For this review, take the finished solid that the model builds, in its own axes (mm). Face numbers are marked on the shaded views. A direction names the side the tool comes from. Coordinates: 2 decimals unless noted, no trailing zeros. Loops run counter-clockwise (first coordinate to the right, second up) from the corner with the lowest first, then second, coordinate; pieces in that order, holes last. Notation, with made-up numbers: M 10,36 L 60,36 A12 cw 60,49 Z; hole C -7,37 d10. An arc over 180 degrees is marked long. Put each result on its own line as item: value.
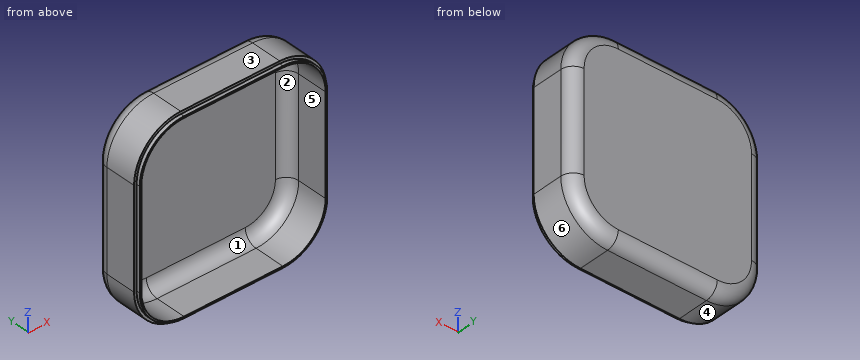
```python
from build123d import *

# Parameters (mm, degrees)
F1_DEPTH = 1.3
F2_DEPTH = 14
F4_DEPTH = 1.2
F5_R     = 4
F6_R     = 4


with BuildPart() as f1:
    # F0 (on Front) → F1 (new body)
    with BuildSketch(Plane.XZ):
        with BuildLine():
            Line((15.9, 30.9), (-15.9, 30.9))
            ThreePointArc((-15.9, 30.9), (-26.506602, 26.506602), (-30.9, 15.9))
            Line((-30.9, 15.9), (-30.9, -15.9))
            ThreePointArc((-30.9, -15.9), (-26.506602, -26.506602), (-15.9, -30.9))
            Line((-15.9, -30.9), (15.9, -30.9))
            ThreePointArc((15.9, -30.9), (26.506602, -26.506602), (30.9, -15.9))
            Line((30.9, -15.9), (30.9, 15.9))
            ThreePointArc((30.9, 15.9), (26.506602, 26.506602), (15.9, 30.9))
        make_face()
        with BuildLine():
            ThreePointArc((-29.6, 15.9), (-25.587363, 25.587363), (-15.9, 29.6))
            Line((-15.9, 29.6), (15.9, 29.6))
            ThreePointArc((15.9, 29.6), (25.587363, 25.587363), (29.6, 15.9))
            Line((29.6, 15.9), (29.6, -15.9))
            ThreePointArc((29.6, -15.9), (25.587363, -25.587363), (15.9, -29.6))
            Line((15.9, -29.6), (-15.9, -29.6))
            ThreePointArc((-15.9, -29.6), (-25.587363, -25.587363), (-29.6, -15.9))
            Line((-29.6, -15.9), (-29.6, 15.9))
        make_face(mode=Mode.SUBTRACT)
        with BuildLine():
            Line((15.9, 29.6), (-15.9, 29.6))
            ThreePointArc((-15.9, 29.6), (-25.587363, 25.587363), (-29.6, 15.9))
            Line((-29.6, 15.9), (-29.6, -15.9))
            ThreePointArc((-29.6, -15.9), (-25.587363, -25.587363), (-15.9, -29.6))
            Line((-15.9, -29.6), (15.9, -29.6))
            ThreePointArc((15.9, -29.6), (25.587363, -25.587363), (29.6, -15.9))
            Line((29.6, -15.9), (29.6, 15.9))
            ThreePointArc((29.6, 15.9), (25.587363, 25.587363), (15.9, 29.6))
        make_face()
    extrude(amount=F1_DEPTH)

    # F0 (on Front) → F2 (join)
    with BuildSketch(Plane.XZ):
        with BuildLine():
            Line((15.9, 30.9), (-15.9, 30.9))
            ThreePointArc((-15.9, 30.9), (-26.506602, 26.506602), (-30.9, 15.9))
            Line((-30.9, 15.9), (-30.9, -15.9))
            ThreePointArc((-30.9, -15.9), (-26.506602, -26.506602), (-15.9, -30.9))
            Line((-15.9, -30.9), (15.9, -30.9))
            ThreePointArc((15.9, -30.9), (26.506602, -26.506602), (30.9, -15.9))
            Line((30.9, -15.9), (30.9, 15.9))
            ThreePointArc((30.9, 15.9), (26.506602, 26.506602), (15.9, 30.9))
        make_face()
        with BuildLine():
            ThreePointArc((-29.6, 15.9), (-25.587363, 25.587363), (-15.9, 29.6))
            Line((-15.9, 29.6), (15.9, 29.6))
            ThreePointArc((15.9, 29.6), (25.587363, 25.587363), (29.6, 15.9))
            Line((29.6, 15.9), (29.6, -15.9))
            ThreePointArc((29.6, -15.9), (25.587363, -25.587363), (15.9, -29.6))
            Line((15.9, -29.6), (-15.9, -29.6))
            ThreePointArc((-15.9, -29.6), (-25.587363, -25.587363), (-29.6, -15.9))
            Line((-29.6, -15.9), (-29.6, 15.9))
        make_face(mode=Mode.SUBTRACT)
    extrude(amount=F2_DEPTH)

    # F3 (on face) → F4 (join)
    with BuildSketch(Plane.XZ.offset(14)):
        with BuildLine():
            Line((15.9, 30.1), (-15.9, 30.1))
            ThreePointArc((-15.9, 30.1), (-25.940916, 25.940916), (-30.1, 15.9))
            Line((-30.1, 15.9), (-30.1, -15.9))
            ThreePointArc((-30.1, -15.9), (-25.940916, -25.940916), (-15.9, -30.1))
            Line((-15.9, -30.1), (15.9, -30.1))
            ThreePointArc((15.9, -30.1), (25.940916, -25.940916), (30.1, -15.9))
            Line((30.1, -15.9), (30.1, 15.9))
            ThreePointArc((30.1, 15.9), (25.940916, 25.940916), (15.9, 30.1))
        make_face()
        with BuildLine():
            Line((15.9, -29.6), (-15.9, -29.6))
            ThreePointArc((-15.9, -29.6), (-25.587363, -25.587363), (-29.6, -15.9))
            Line((-29.6, -15.9), (-29.6, 15.9))
            ThreePointArc((-29.6, 15.9), (-25.587363, 25.587363), (-15.9, 29.6))
            Line((-15.9, 29.6), (15.9, 29.6))
            ThreePointArc((15.9, 29.6), (25.587363, 25.587363), (29.6, 15.9))
            Line((29.6, 15.9), (29.6, -15.9))
            ThreePointArc((29.6, -15.9), (25.587363, -25.587363), (15.9, -29.6))
        make_face(mode=Mode.SUBTRACT)
    extrude(amount=F4_DEPTH)

    # F5
    f5_edges = [f1.edges().sort_by_distance(p)[0] for p in [
        (-25.587363, -1.3, -25.587363),
    ]]
    fillet(f5_edges, radius=F5_R)

    # F6
    f6_edges = [f1.edges().sort_by_distance(p)[0] for p in [
        (0, 0, 30.9),
        (-26.506602, 0, 26.506602),
        (-30.9, 0, 0),
        (-26.506602, 0, -26.506602),
        (0, 0, -30.9),
        (26.506602, 0, -26.506602),
        (30.9, 0, 0),
        (26.506602, 0, 26.506602),
    ]]
    fillet(f6_edges, radius=F6_R)


solid = f1.part
```
(1) Add section B-B (x = 7). Write out the cut boundary in (y, z).
Determined:
outline: M -15.2,-30.1 L -14,-30.1 L -14,-30.9 L -4,-30.9 A4 ccw 0,-26.9 L 0,26.9 A4 ccw -4,30.9 L -14,30.9 L -14,30.1 L -15.2,30.1 L -15.2,29.6 L -5.3,29.6 A4 cw -1.3,25.6 L -1.3,-25.6 A4 cw -5.3,-29.6 L -15.2,-29.6 Z
(2) Tool access review of the marked faces 5 and 6: name each direction out of +Z, -Z, +X, -X, +Y, -Y from which nothing blocks a thin tool from reaching the whole face with its end or side.
Determined:
face 5: -Y
face 6: -Z, +X, +Y, -Y
(3) For pin 1 (1.5 mm diameter, centred on y = -7, z = -17.5, fed in from -X); pin 2 (12 mm diameter, centred on x = 17, z = 10.5, fed in from -Y), all flat-tipped, find the tip position at first contact; note any pin that passes through.
Determined:
pin 1: stops at x = -30.88
pin 2: stops at y = -1.3
(4) Draft analysis for pull direction X (two halves, no side actions). For the marked faces 1, 2, 3 and 4, state which applies: +X half, -X half, draft (parallel to the pull), parting line (faces both ways), or undercut.
Determined:
face 1: undercut
face 2: undercut
face 3: draft
face 4: -X half
(5) Wall thickness on line 1 along X through (y, z) = (-10.75, -10); line 2 along Y through (x, z) = (-7, -15): over which ranges is each line inside the solid? List them lowest first. Write a range as [from, to].
Determined:
line 1: x = [-30.9, -29.6], [29.6, 30.9]
line 2: y = [-1.3, 0]
(6) Add section A-A (y = -6.75). Write out the cut boundary in (x, z), plus the area to 3 significant figures.
Determined:
outline: M -30.9,-15.9 A15 ccw -15.9,-30.9 L 15.9,-30.9 A15 ccw 30.9,-15.9 L 30.9,15.9 A15 ccw 15.9,30.9 L -15.9,30.9 A15 ccw -30.9,15.9 Z; hole M -29.6,-15.9 A13.7 ccw -15.9,-29.6 L 15.9,-29.6 A13.7 ccw 29.6,-15.9 L 29.6,15.9 A13.7 ccw 15.9,29.6 L -15.9,29.6 A13.7 ccw -29.6,15.9 Z
area: 283 mm^2
(7) Add section C-C (z = 1). Write out the cut boundary in (x, y), plus the area to 3 significant figures.
Determined:
outline: M -30.9,-14 L -30.1,-14 L -30.1,-15.2 L -29.6,-15.2 L -29.6,-5.3 A4 cw -25.6,-1.3 L 25.6,-1.3 A4 cw 29.6,-5.3 L 29.6,-15.2 L 30.1,-15.2 L 30.1,-14 L 30.9,-14 L 30.9,-4 A4 ccw 26.9,0 L -26.9,0 A4 ccw -30.9,-4 Z
area: 115 mm^2
